Here's the drawing with two shaded views (mm, measured from the low corner). I have some questions. Give positions to 0.01 mm unless a question says otherwise; leave off trailing zeros. Loops run counter-clockwise (first coordinate to the right, second up) from the corner with the lowest first, then second, coordinate; pieces in that order, holes last. Notation, with made-up numbers: M 67,2 L 74,2 A11 cw 74,14 Z; hole C 66.25,65 d2. An arc over 180 degrees is marked long. Use CSV: the item, a comma, the result in double quotes.
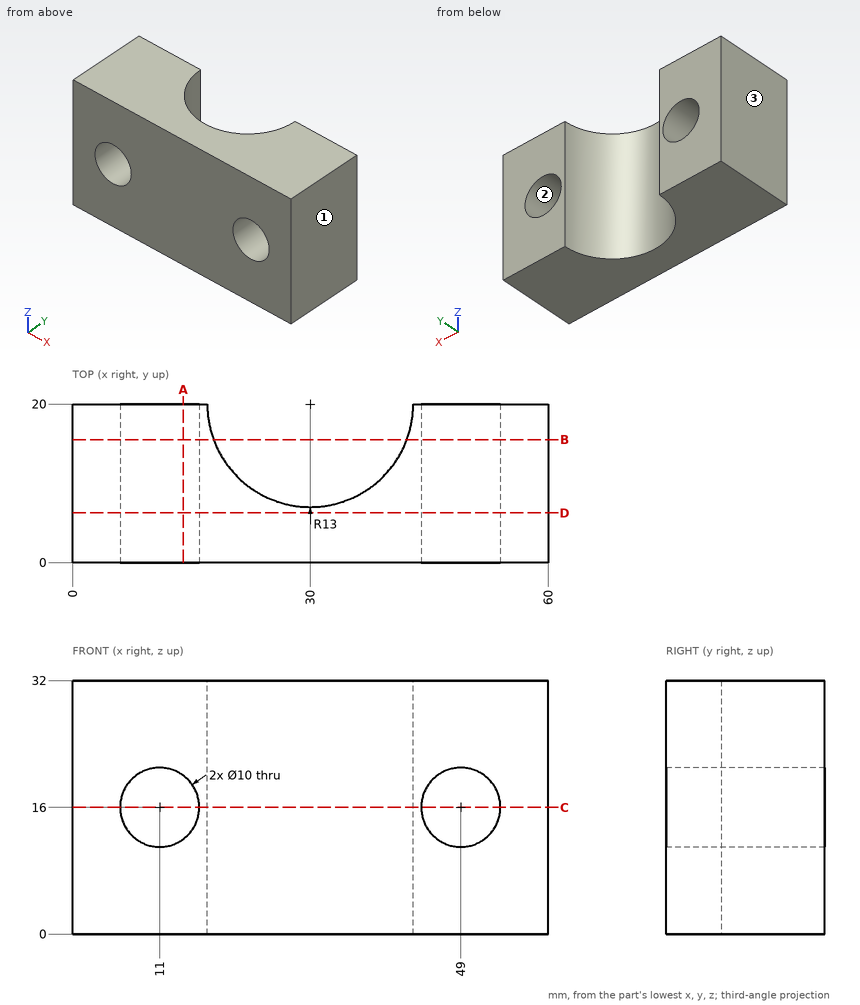
1. I want a section at B-B, the plane y = 15.5. List the corners of the cut face in (x, z) for me, then the cut area to 3 significant figures.
Outcome:
outline,"M 0,0 L 17.8,0 L 17.8,32 L 0,32 Z; M 42.2,0 L 60,0 L 60,32 L 42.2,32 Z; hole C 11,16 d10; hole C 49,16 d10"
area,"982 mm2"
2. I want a section at D-D, the plane y = 6.25. List the corners of the cut face in (x, z) for me, then the cut area to 3 significant figures.
Outcome:
outline,"M 0,0 L 60,0 L 60,32 L 0,32 Z; hole C 11,16 d10; hole C 49,16 d10"
area,"1,760 mm2"
3. If we mould it in two halves opening along X, with no side actions, what happens to the marked faces 1, 2 and 3? For each: +X half, -X half, draft (parallel to the pull), parting line (faces both ways), or undercut.
Outcome:
face 1,"+X half"
face 2,"undercut"
face 3,"-X half"
4. Please list where these lines run through material, in increasing order: line 1 (X direction, y = 13, z = 19); line 2 (X direction, y = 16, z = 12.5); line 3 (X direction, y = 6.5, z = 19).
Outcome:
line 1,"0 to 7, 15 to 19.05, 40.95 to 45, 53 to 60"
line 2,"0 to 7.43, 14.57 to 17.63, 42.37 to 45.43, 52.57 to 60"
line 3,"0 to 7, 15 to 45, 53 to 60"
5. I'm going to push flat-ended pins straight in: pin 1 Ø2 at (x, y) = (36, 9) entering from -Z; pin 2 Ø8 at (x, z) = (49, 16) entering from +Y; pin 3 Ø1 at (x, z) = (34, 15) entering from +Y. Where does each tip first touch, or does it pass through?
Outcome:
pin 1,"z = 0"
pin 2,"through"
pin 3,"y = 7.8"
6. I want a section at A-A, the plane x = 14. List the corners of the cut face in (y, z) for me, then the cut area to 3 significant figures.
Outcome:
outline,"M 0,0 L 20,0 L 20,12 L 0,12 Z; M 0,20 L 20,20 L 20,32 L 0,32 Z"
area,"480 mm2"
7. I want a section at C-C, the plane z = 16. List the corners of the cut face in (x, y) for me, then the cut area to 3 significant figures.
Outcome:
outline,"M 0,0 L 6,0 L 6,20 L 0,20 Z; M 16,0 L 44,0 L 44,20 L 43,20 A13 cw 17,20 L 16,20 Z; M 54,0 L 60,0 L 60,20 L 54,20 Z"
area,"535 mm2"
